from build123d import *

# Parameters (mm, degrees)
SKETCH1_W               = 50
SKETCH1_H               = 110
BOSS_EXTRUDE1_DEPTH     = 2
SKETCH2_W               = 50
SKETCH2_H               = 110
SKETCH2_W_2             = 46
SKETCH2_H_2             = 106
BOSS_EXTRUDE3_DEPTH     = 11
SKETCH3_R               = 1.2
BOSS_EXTRUDE4_DEPTH     = 11
SKETCH4_W               = 52
SKETCH4_H               = 112
SKETCH4_W_2             = 50
SKETCH4_H_2             = 110
EXTRUDE_THIN1_DEPTH     = 13
FILLET2_R               = 2
EXTRUDE_THIN3_DEPTH     = 3
SKETCH6_R               = 1.8
BOSS_EXTRUDE5_DEPTH     = 2.8
SKETCH8_W               = 8
SKETCH8_H               = 3.6
CUT_EXTRUDE2_DEPTH      = 12.8
SKETCH11_W              = 13.1
SKETCH11_H              = 5.8
CUT_EXTRUDE5_DEPTH      = 3
SKETCH13_W              = 108
SKETCH13_H              = 3
CUT_EXTRUDE6_DEPTH      = 70
CUT_EXTRUDE6_DEPTH_BACK = 40
SKETCH14_W              = 48
SKETCH14_H              = 3
CUT_EXTRUDE7_DEPTH      = 160
CUT_EXTRUDE7_DEPTH_BACK = 40
SKETCH15_W              = 66.867567733
SKETCH15_H              = 122.152543676
CUT_EXTRUDE8_DEPTH      = 40
SKETCH16_W              = 37.40524021
SKETCH16_H              = 102.153015582
CUT_EXTRUDE9_DEPTH      = 5
CUT_EXTRUDE_THIN2_DEPTH = 55
SKETCH18_W              = 13.9
SKETCH18_H              = 6.6
CUT_EXTRUDE10_DEPTH     = 2


with BuildPart() as part:
    # Sketch1 → Boss-Extrude1 (new body)
    with BuildSketch(Plane(origin=(0, 0, 0), x_dir=(1, 0, 0), z_dir=(0, 1, 0))):
        with Locations((-52.022587269, -1.919917864)):
            Rectangle(SKETCH1_W, SKETCH1_H)
    extrude(amount=BOSS_EXTRUDE1_DEPTH)

    # Sketch2 → Boss-Extrude3 (add)
    with BuildSketch(Plane(origin=(0, 2, 0), x_dir=(1, 0, 0), z_dir=(0, 1, 0))):
        with Locations((-52.022587269, -1.919917864)):
            Rectangle(SKETCH2_W, SKETCH2_H)
        with Locations((-52.022587269, -1.919917864)):
            Rectangle(SKETCH2_W_2, SKETCH2_H_2, mode=Mode.SUBTRACT)
    extrude(amount=BOSS_EXTRUDE3_DEPTH)

    # Sketch3 → Boss-Extrude4 (add)
    with BuildSketch(Plane(origin=(0, 2, 0), x_dir=(1, 0, 0), z_dir=(0, 1, 0))):
        with Locations((-31.022587269, 42.380082136)):
            Circle(SKETCH3_R)
        with Locations((-31.022587269, -52.919917864)):
            Circle(SKETCH3_R)
        with Locations((-56.322587269, 42.380082136)):
            Circle(SKETCH3_R)
        with Locations((-56.322587269, -52.919917864)):
            Circle(SKETCH3_R)
    extrude(amount=BOSS_EXTRUDE4_DEPTH)

    # Sketch4 → Extrude-Thin1 (add)
    with BuildSketch(Plane(origin=(0, 13, 0), x_dir=(1, 0, 0), z_dir=(0, 1, 0))):
        with Locations((-52.022587269, -1.919917864)):
            Rectangle(SKETCH4_W, SKETCH4_H)
        with Locations((-52.022587269, -1.919917864)):
            Rectangle(SKETCH4_W_2, SKETCH4_H_2, mode=Mode.SUBTRACT)
    extrude(amount=-EXTRUDE_THIN1_DEPTH)

    # Fillet2
    fillet2_edges = [part.edges().sort_by_distance(p)[0] for p in [
        (-26.022587269, 6.5, -54.080082136),
        (-26.022587269, 6.5, 57.919917864),
        (-78.022587269, 6.5, 57.919917864),
        (-78.022587269, 6.5, -54.080082136),
    ]]
    fillet(fillet2_edges, radius=FILLET2_R)

    # Sketch5 → Extrude-Thin3 (add)
    with BuildSketch(Plane(origin=(0, 13, 0), x_dir=(1, 0, 0), z_dir=(0, 1, 0))):
        with BuildLine():
            Line((-28.022587269, 54.080082136), (-76.022587269, 54.080082136))
            ThreePointArc((-76.022587269, 54.080082136), (-77.436800831, 53.494295698), (-78.022587269, 52.080082136))
            Line((-78.022587269, 52.080082136), (-78.022587269, -55.919917864))
            ThreePointArc((-78.022587269, -55.919917864), (-77.436800831, -57.334131427), (-76.022587269, -57.919917864))
            Line((-76.022587269, -57.919917864), (-28.022587269, -57.919917864))
            ThreePointArc((-28.022587269, -57.919917864), (-26.608373707, -57.334131427), (-26.022587269, -55.919917864))
            Line((-26.022587269, -55.919917864), (-26.022587269, 52.080082136))
            ThreePointArc((-26.022587269, 52.080082136), (-26.608373707, 53.494295698), (-28.022587269, 54.080082136))
        make_face()
        with BuildLine():
            Line((-28.022587269, 52.880082136), (-76.022587269, 52.880082136))
            ThreePointArc((-76.022587269, 52.880082136), (-76.588272694, 52.64576756), (-76.822587269, 52.080082136))
            Line((-76.822587269, 52.080082136), (-76.822587269, -55.919917864))
            ThreePointArc((-76.822587269, -55.919917864), (-76.588272694, -56.485603289), (-76.022587269, -56.719917864))
            Line((-76.022587269, -56.719917864), (-28.022587269, -56.719917864))
            ThreePointArc((-28.022587269, -56.719917864), (-27.456901844, -56.485603289), (-27.222587269, -55.919917864))
            Line((-27.222587269, -55.919917864), (-27.222587269, 52.080082136))
            ThreePointArc((-27.222587269, 52.080082136), (-27.456901844, 52.64576756), (-28.022587269, 52.880082136))
        make_face(mode=Mode.SUBTRACT)
    extrude(amount=EXTRUDE_THIN3_DEPTH)

    # Sketch6 → Boss-Extrude5 (add)
    with BuildSketch(Plane(origin=(0, 2, 0), x_dir=(1, 0, 0), z_dir=(0, 1, 0))):
        with Locations((-56.322587269, -52.919917864)):
            Circle(SKETCH6_R)
        with Locations((-31.022587269, -52.919917864)):
            Circle(SKETCH6_R)
        with Locations((-56.322587269, 42.380082136)):
            Circle(SKETCH6_R)
        with Locations((-31.022587269, 42.380082136)):
            Circle(SKETCH6_R)
    extrude(amount=BOSS_EXTRUDE5_DEPTH)

    # Sketch8 → Cut-Extrude2 (cut)
    with BuildSketch(Plane(origin=(-26.022587269, 0, 0), x_dir=(0, 0, -1), z_dir=(1, 0, 0))):
        with Locations((-44.619917864, 3.8)):
            Rectangle(SKETCH8_W, SKETCH8_H)
    extrude(amount=-CUT_EXTRUDE2_DEPTH, mode=Mode.SUBTRACT)

    # Sketch11 → Cut-Extrude5 (cut)
    with BuildSketch(Plane.ZY.offset(78.022587269)):
        with Locations((-43.530082136, 4.9)):
            Rectangle(SKETCH11_W, SKETCH11_H)
    extrude(amount=-CUT_EXTRUDE5_DEPTH, mode=Mode.SUBTRACT)

    # Sketch13 → Cut-Extrude6 (cut, two sides)
    with BuildSketch(Plane(origin=(-76.822587269, 0, 0), x_dir=(0, 0, -1), z_dir=(1, 0, 0))) as cut_extrude6_sk:
        with Locations((-1.919917864, 14.5)):
            Rectangle(SKETCH13_W, SKETCH13_H)
    extrude(amount=CUT_EXTRUDE6_DEPTH, mode=Mode.SUBTRACT)
    extrude(cut_extrude6_sk.sketch, amount=-CUT_EXTRUDE6_DEPTH_BACK, mode=Mode.SUBTRACT)

    # Sketch14 → Cut-Extrude7 (cut, two sides)
    with BuildSketch(Plane.XY.offset(-52.880082136)) as cut_extrude7_sk:
        with Locations((-52.022587269, 14.5)):
            Rectangle(SKETCH14_W, SKETCH14_H)
    extrude(amount=CUT_EXTRUDE7_DEPTH, mode=Mode.SUBTRACT)
    extrude(cut_extrude7_sk.sketch, amount=-CUT_EXTRUDE7_DEPTH_BACK, mode=Mode.SUBTRACT)

    # Sketch15 → Cut-Extrude8 (cut)
    with BuildSketch(Plane(origin=(0, 13, 0), x_dir=(1, 0, 0), z_dir=(0, 1, 0))):
        with Locations((-54.115240408, -0.313928246)):
            Rectangle(SKETCH15_W, SKETCH15_H)
    extrude(amount=CUT_EXTRUDE8_DEPTH, mode=Mode.SUBTRACT)

    # Sketch16 → Cut-Extrude9 (cut)
    with BuildSketch(Plane(origin=(0, 13, 0), x_dir=(1, 0, 0), z_dir=(0, 1, 0))):
        with Locations((-47.725207374, -3.843410073)):
            Rectangle(SKETCH16_W, SKETCH16_H)
    extrude(amount=-CUT_EXTRUDE9_DEPTH, mode=Mode.SUBTRACT)

    # Sketch17 → Cut-Extrude-Thin2 (cut)
    with BuildSketch(Plane(origin=(0, 13, 0), x_dir=(1, 0, 0), z_dir=(0, 1, 0))):
        with BuildLine():
            Line((-97.022587269, 52.080082136), (-97.022587269, -55.919917864))
            ThreePointArc((-97.022587269, -55.919917864), (-90.871829674, -70.769160269), (-76.022587269, -76.919917864))
            Line((-76.022587269, -76.919917864), (-28.022587269, -76.919917864))
            ThreePointArc((-28.022587269, -76.919917864), (-13.173344864, -70.769160269), (-7.022587269, -55.919917864))
            Line((-7.022587269, -55.919917864), (-7.022587269, 52.080082136))
            ThreePointArc((-7.022587269, 52.080082136), (-13.173344864, 66.92932454), (-28.022587269, 73.080082136))
            Line((-28.022587269, 73.080082136), (-76.022587269, 73.080082136))
            ThreePointArc((-76.022587269, 73.080082136), (-90.871829674, 66.92932454), (-97.022587269, 52.080082136))
        make_face()
        with BuildLine():
            Line((-77.022587269, 52.080082136), (-77.022587269, -55.919917864))
            ThreePointArc((-77.022587269, -55.919917864), (-76.72969405, -56.627024646), (-76.022587269, -56.919917864))
            Line((-76.022587269, -56.919917864), (-28.022587269, -56.919917864))
            ThreePointArc((-28.022587269, -56.919917864), (-27.315480488, -56.627024646), (-27.022587269, -55.919917864))
            Line((-27.022587269, -55.919917864), (-27.022587269, 52.080082136))
            ThreePointArc((-27.022587269, 52.080082136), (-27.315480488, 52.787188917), (-28.022587269, 53.080082136))
            Line((-28.022587269, 53.080082136), (-76.022587269, 53.080082136))
            ThreePointArc((-76.022587269, 53.080082136), (-76.72969405, 52.787188917), (-77.022587269, 52.080082136))
        make_face(mode=Mode.SUBTRACT)
    extrude(amount=-CUT_EXTRUDE_THIN2_DEPTH, mode=Mode.SUBTRACT)

    # Sketch18 → Cut-Extrude10 (cut)
    with BuildSketch(Plane.ZY.offset(77.022587269)):
        with Locations((-43.130082136, 5.3)):
            Rectangle(SKETCH18_W, SKETCH18_H)
    extrude(amount=-CUT_EXTRUDE10_DEPTH, mode=Mode.SUBTRACT)


solid = part.part
Verification items for the finished model (mm, model axes). A direction names the side the tool comes from. Coordinates: 2 decimals unless noted, no trailing zeros. Order: outer loops, then holes, each group sorted by start corner. A loop starts at its lowest first (then second) coordinate and runs counter-clockwise, first axis right, second up. Notation, with made-up numbers: M 23.25,45 L 62.25,45 A21 cw 62.25,81 Z; hole C 29,84.25 d9. An arc over 180 degrees is marked long. One line per item, written item: value. Start each with the question number.
Item 1: Scan lines: probe 1 along Z at (x, y) = (-49.5, 8); probe 2 along X at (y, z) = (9.5, -30); probe 3 along Y at (x, z) = (-63, 33.5). Record each from-to range of solid material in increasing order.
Item 2: Access from +Z, -Z, +X, -X, +Y, -Y to the whole of each face (thin tool, end or side, straight path). Record for faces 1 (the flat face through (-28, 5.6, 45)), 2 (the flat face through (-76, 5, -36.18)), 3 (the flat face through (-77.023, 7, 1)), 4 (the flat face through (-31, 8, -42)), 5 (the flat face through (-31, 8, 53)).
Item 3: Sectioned sample at C-C (z = 20). Enter the section's corners in (x, y), then the cut area to 3 significant figures.
Item 4: Sectioned sample at B-B (x = -50.5). Enter the section's corners in (y, z), then the cut area to 3 significant figures.
Item 5: Mould release check, pull along Z, two halves, no side actions. Record for faces 6 (the flat face through (-52, 7, -53.08)), 7 (the cylindrical face through (-31.257, 3.38, -44.165)), 8 (the cylindrical face through (-31.975, 6.378, -41.65)), 9 (the flat face through (-76, 13, -15)): released by +Z, released by -Z, zero draft, split by the parting line, or undercut.
Item 6: Gauge pin test, flat ends, axial feed: pin 1 (0.7 mm diameter, centred on x = -31, z = 52.5, fed in from +Y); pin 2 (4 mm diameter, centred on x = -58.5, z = -33, fed in from +Y); pin 3 (1 mm diameter, centred on x = -75.5, z = -42, fed in from -Y). Record the tip position at first contact, or that the pin passes through.
Item 7: Sectioned sample at A-A (y = 10.75). Enter the section's corners in (x, z).
Conclusion:
1. probe 1: z = -53.08 to -51.08, 54.92 to 56.92
1. probe 2: x = -77.02 to -75.02, -29.02 to -27.02
1. probe 3: y = 0 to 2
2. face 1: +X
2. face 2: -X
2. face 3: +Z, -Z, -X, +Y, -Y
2. face 4: -X, +Y
2. face 5: +Y
3. outline: M -77.02,0 L -27.02,0 L -27.02,13 L -29.02,13 L -29.02,2 L -75.02,2 L -75.02,13 L -77.02,13 Z
3. area: 144 mm^2
4. outline: M 0,-53.08 L 13,-53.08 L 13,-51.08 L 2,-51.08 L 2,54.92 L 13,54.92 L 13,56.92 L 0,56.92 Z
4. area: 264 mm^2
5. face 6: released by -Z
5. face 7: undercut
5. face 8: undercut
5. face 9: zero draft
6. pin 1: stops at y = 8
6. pin 2: stops at y = 2
6. pin 3: stops at y = 0
7. outline: M -77.02,-52.08 A1 ccw -76.02,-53.08 L -28.02,-53.08 A1 ccw -27.02,-52.08 L -27.02,55.92 A1 ccw -28.02,56.92 L -76.02,56.92 A1 ccw -77.02,55.92 Z; hole M -75.02,-51.08 L -29.02,-51.08 L -29.02,54.92 L -75.02,54.92 Z
